Check sheet for the drawn part. Datum: minimum x, y, z corner. Units: mm. Coordinates: 2 decimals unless noted, no trailing zeros. Write each loop counter-clockwise with the first axis right and the second up, starting at its lowest first coordinate (ties: lowest second). Pieces come first, ordered by that corner, then holes. Notation, with made-up numbers: M 87.5,21.5 L 101.5,21.5 A6 ccw 101.5,25.5 Z; hole C -5.5,53 d3. An arc over 180 degrees is marked long. Write item = value, one per line. Start each with the question number.
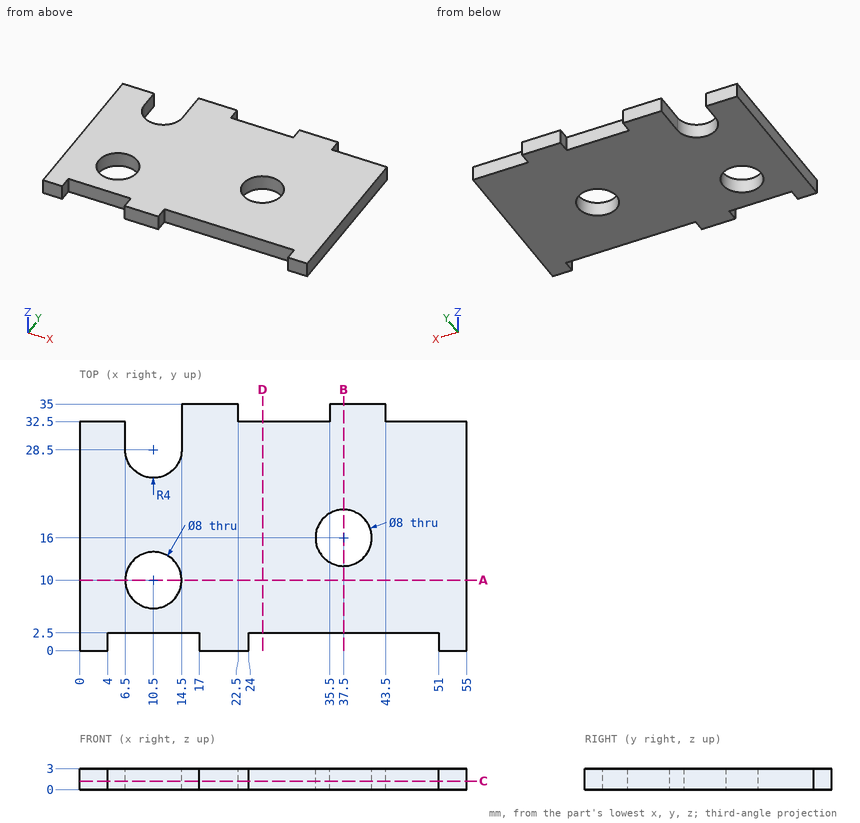
Q1. Cross-section at C-C on z = 1.2. Enter the section's corners in (x, y).
Q2. Cross-section at A-A on y = 10. Enter the section's corners in (x, z), and give its area (3 significant figures).
Q3. Scan lines: L1, parallel to X at y = 32, z = 2.8; L2, parallel to Y at x = 10.5, z = 2.05; L3, parallel to Y at x = 37.5, z = 2.05. Record each from-to range of solid material in increasing order.
Q4. Cross-section at D-D on x = 26. Enter the section's corners in (y, z), and give its area (3 significant figures).
Q5. Gauge pin test, flat ends, axial feed: pin 1 (1.5 mm diameter, centred on x = 51, z = 2, fed in from +Y); pin 2 (0.9 mm diameter, centred on x = 8.5, z = 2, fed in from -Y). Record the tip position at first contact, or that the pin passes through.
Q6. Cross-section at B-B on x = 37.5. Enter the section's corners in (y, z).
Values found:
q1.outline = M 0,0 L 4,0 L 4,2.5 L 17,2.5 L 17,0 L 24,0 L 24,2.5 L 51,2.5 L 51,0 L 55,0 L 55,32.5 L 43.5,32.5 L 43.5,35 L 35.5,35 L 35.5,32.5 L 22.5,32.5 L 22.5,35 L 14.5,35 L 14.5,28.5 A4 cw 6.5,28.5 L 6.5,32.5 L 0,32.5 Z; hole C 10.5,10 d8; hole C 37.5,16 d8
q2.outline = M 0,0 L 6.5,0 L 6.5,3 L 0,3 Z; M 14.5,0 L 55,0 L 55,3 L 14.5,3 Z
q2.area = 141 mm²
q3.L1 = 0 to 6.5, 14.5 to 55
q3.L2 = 2.5 to 6, 14 to 24.5
q3.L3 = 2.5 to 12, 20 to 35
q4.outline = M 2.5,0 L 32.5,0 L 32.5,3 L 2.5,3 Z
q4.area = 90.0 mm²
q5.pin_1 = 32.5
q5.pin_2 = 2.5
q6.outline = M 2.5,0 L 12,0 L 12,3 L 2.5,3 Z; M 20,0 L 35,0 L 35,3 L 20,3 Z
